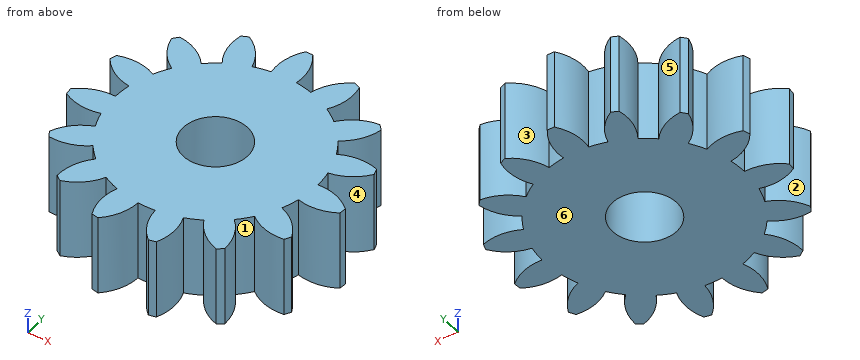
from build123d import *

# Parameters (mm, degrees)
MODEL_R             = 2
BOSS_EXTRUDE1_DEPTH = 5


with BuildPart() as part:
    # Model → Boss-Extrude1 (new body)
    with BuildSketch(Plane.XY):
        with BuildLine():
            ThreePointArc((455.213810884, 475.737053866), (455.579522306, 476.123501007), (455.911034715, 476.539656939))
            ThreePointArc((455.911034715, 476.539656939), (456.985627664, 475.992517671), (458.188848778, 475.912703304))
            ThreePointArc((458.188848778, 475.912703304), (458.297616539, 476.103235845), (458.401430664, 476.296512079))
            ThreePointArc((458.401430664, 476.296512079), (457.695483937, 477.274137059), (456.66162305, 477.894816565))
            ThreePointArc((456.66162305, 477.894816565), (456.838534846, 478.396601831), (456.972120634, 478.911617437))
            ThreePointArc((456.972120634, 478.911617437), (458.176351731, 478.848857172), (459.308012342, 479.265337237))
            ThreePointArc((459.308012342, 479.265337237), (459.329880069, 479.483637208), (459.346106466, 479.702428842))
            ThreePointArc((459.346106466, 479.702428842), (458.303556137, 480.3083993), (457.106624121, 480.454909137))
            ThreePointArc((457.106624121, 480.454909137), (457.064146634, 480.985269298), (456.976707605, 481.5100937))
            ThreePointArc((456.976707605, 481.5100937), (458.102354353, 481.942564259), (458.96678006, 482.783325568))
            ThreePointArc((458.96678006, 482.783325568), (458.897966625, 482.991646922), (458.823799602, 483.198122895))
            ThreePointArc((458.823799602, 483.198122895), (457.624912095, 483.327661034), (456.471869369, 482.974668319))
            ThreePointArc((456.471869369, 482.974668319), (456.217347342, 483.441899284), (455.9240025, 483.885785577))
            ThreePointArc((455.9240025, 483.885785577), (456.776430349, 484.73870887), (457.224154095, 485.858376156))
            ThreePointArc((457.224154095, 485.858376156), (457.076557966, 486.020698236), (456.924821674, 486.179156978))
            ThreePointArc((456.924821674, 486.179156978), (455.776895531, 485.809864476), (454.867113658, 485.018404858))
            ThreePointArc((454.867113658, 485.018404858), (454.444556262, 485.341718149), (453.996027593, 485.627914358))
            ThreePointArc((453.996027593, 485.627914358), (454.427844026, 486.753812201), (454.381450307, 487.958784817))
            ThreePointArc((454.381450307, 487.958784817), (454.180592196, 488.047040662), (453.977523219, 488.130083216))
            ThreePointArc((453.977523219, 488.130083216), (453.079045297, 487.325814102), (452.569833828, 486.232738138))
            ThreePointArc((452.569833828, 486.232738138), (452.052305076, 486.35622995), (451.526147262, 486.435250151))
            ThreePointArc((451.526147262, 486.435250151), (451.462687294, 487.639444578), (450.930198006, 488.721371813))
            ThreePointArc((450.930198006, 488.721371813), (450.710808105, 488.720301185), (450.491518914, 488.713568739))
            ThreePointArc((450.491518914, 488.713568739), (449.997844209, 487.613388449), (449.977250433, 486.407698904))
            ThreePointArc((449.977250433, 486.407698904), (449.454235747, 486.31001638), (448.941426255, 486.168197264))
            ThreePointArc((448.941426255, 486.168197264), (448.393662691, 487.242472118), (447.467150069, 488.014278923))
            ThreePointArc((447.467150069, 488.014278923), (447.267162884, 487.924066944), (447.069570573, 487.828723599))
            ThreePointArc((447.069570573, 487.828723599), (447.066059926, 486.622863301), (447.537644694, 485.51303485))
            ThreePointArc((447.537644694, 485.51303485), (447.099578065, 485.211068187), (446.688786314, 484.872931566))
            ThreePointArc((446.688786314, 484.872931566), (445.751432451, 485.631534965), (444.591098944, 485.959768933))
            ThreePointArc((444.591098944, 485.959768933), (444.445094078, 485.796014074), (444.303364151, 485.62854556))
            ThreePointArc((444.303364151, 485.62854556), (444.790624586, 484.525509454), (445.672846607, 483.703441519))
            ThreePointArc((445.672846607, 483.703441519), (445.395473735, 483.249403495), (445.157729351, 482.773416263))
            ThreePointArc((445.157729351, 482.773416263), (443.992862186, 483.085178789), (442.79934, 482.913085284))
            ThreePointArc((442.79934, 482.913085284), (442.732563019, 482.704102247), (442.67120187, 482.493465393))
            ThreePointArc((442.67120187, 482.493465393), (443.56498163, 481.683978441), (444.705296702, 481.291814037))
            ThreePointArc((444.705296702, 481.291814037), (444.636577876, 480.764211952), (444.612989023, 480.232676626))
            ThreePointArc((444.612989023, 480.232676626), (443.422024673, 480.043691705), (442.401684635, 479.401027258))
            ThreePointArc((442.401684635, 479.401027258), (442.425681887, 479.182951108), (442.455299415, 478.965566939))
            ThreePointArc((442.455299415, 478.965566939), (443.60105586, 478.589596791), (444.802293147, 478.695144705))
            ThreePointArc((444.802293147, 478.695144705), (444.954110477, 478.185205752), (445.148755882, 477.690029618))
            ThreePointArc((445.148755882, 477.690029618), (444.137622902, 477.03297446), (443.466891075, 476.030861592))
            ThreePointArc((443.466891075, 476.030861592), (443.577513216, 475.841399678), (443.692988281, 475.654855892))
            ThreePointArc((443.692988281, 475.654855892), (444.892609713, 475.777411201), (445.947064377, 476.36242124))
            ThreePointArc((445.947064377, 476.36242124), (446.293167267, 475.958318498), (446.67239097, 475.585122008))
            ThreePointArc((446.67239097, 475.585122008), (446.015923439, 474.573607419), (445.810775449, 473.385320549))
            ThreePointArc((445.810775449, 473.385320549), (445.988894907, 473.257232556), (446.170260821, 473.133784268))
            ThreePointArc((446.170260821, 473.133784268), (447.216321796, 473.733674108), (447.941669045, 474.696992722))
            ThreePointArc((447.941669045, 474.696992722), (448.422213161, 474.468599225), (448.92044394, 474.281911443))
            ThreePointArc((448.92044394, 474.281911443), (448.732151056, 473.090837485), (449.028058855, 471.921842207))
            ThreePointArc((449.028058855, 471.921842207), (449.242877156, 471.877275714), (449.458774107, 471.838268254))
            ThreePointArc((449.458774107, 471.838268254), (450.170401179, 472.811766221), (450.441221884, 473.986826871))
            ThreePointArc((450.441221884, 473.986826871), (450.973116782, 473.973633929), (451.504206009, 474.005734869))
            ThreePointArc((451.504206009, 474.005734869), (451.816645324, 472.84104905), (452.562443764, 471.893475269))
            ThreePointArc((452.562443764, 471.893475269), (452.776816874, 471.940136226), (452.989914315, 471.992314338))
            ThreePointArc((452.989914315, 471.992314338), (453.244060699, 473.171093791), (453.0135275, 474.354717814))
            ThreePointArc((453.0135275, 474.354717814), (453.504803721, 474.559006608), (453.976921244, 474.804345725))
            ThreePointArc((453.976921244, 474.804345725), (454.736069161, 473.867432804), (455.802802917, 473.305124634))
            ThreePointArc((455.802802917, 473.305124634), (455.979663777, 473.434944938), (456.153115226, 473.569286554))
            ThreePointArc((456.153115226, 473.569286554), (455.905836703, 474.749525816), (455.213810884, 475.737053866))
        make_face()
        with Locations((450.861979287, 480.22164557)):
            Circle(MODEL_R, mode=Mode.SUBTRACT)
    extrude(amount=BOSS_EXTRUDE1_DEPTH)


solid = part.part
Work out the finished part from the listing and answer in its coordinate system (mm). Face numbers are marked on the shaded views. A direction names the side the tool comes from. Give positions to 0.01 mm unless a question says otherwise; leave off trailing zeros. Order: outer loops, then holes, each group sorted by start corner. A loop starts at its lowest first (then second) coordinate and runs counter-clockwise, first axis right, second up. Notation, with made-up numbers: (17.5, -39) -> (22.5, -39) arc R24 cw to (22.5, -6) -> close; hole circle Ø6 at (-10, -1). An arc over 180 degrees is marked (long way). Answer as a JSON object with one key per item and string values. Group by question number.
1. Section A-A on y = 487.5 is taken. Determine the outline of the cut face in (x, z).
2. Section D-D on x = 453.5 is taken. Determine the outline of the cut face in (y, z).
3. Section C-C on y = 480 is taken. Determine the outline of the cut face in (x, z).
4. Flat-ended cylindrical pins translate along their axes: pin 1 Ø2 at (x, z) = (451.5, 2) entering from -Y; pin 2 Ø3 at (x, z) = (446.5, 3) entering from -Y; pin 3 Ø8 at (x, y) = (447, 477.5) entering from -Z. Find the tip coordinate at first contact, or state that the pin passes through.
5. Consider line 1 along Y through (x, z) = (450.75, 3.55); line 2 along X through (y, z) = (473.25, 3.1); line 3 along Y through (x, z) = (444, 0.3). Determine where each line is inside the solid, lowest interval first. Write a range as [from, to].
6. A tool of negligible diameter and unlimited length cuts with its end or side. For the marked faces 1, 2 and 3, from which of +Z, -Z, +X, -X, +Y, -Y can it reach the whole face along a straight path? Write none if from no direction.
7. The mould has two halves that part along X. Classify the marked faces 4, 5 and 6: released by +X, released by -X, zero draft, split by the parting line, or undercut.
8. Section B-B on x = 444 is taken. Determine the outline of the cut face in (y, z), plus the area to 3 significant figures.
Result sheet:
{
 "1": {"outline": "(447.02, 0) -> (448.16, 0) -> (448.16, 5) -> (447.02, 5) -> close; (449.97, 0) -> (451.5, 0) -> (451.5, 5) -> (449.97, 5) -> close; (453.22, 0) -> (454.46, 0) -> (454.46, 5) -> (453.22, 5) -> close"},
 "2": {"outline": "(474.56, 0) -> (487.78, 0) -> (487.78, 5) -> (474.56, 5) -> close"},
 "3": {"outline": "(443.31, 0) -> (448.87, 0) -> (448.87, 5) -> (443.31, 5) -> close; (452.85, 0) -> (458.95, 0) -> (458.95, 5) -> (452.85, 5) -> close"},
 "4": {"pin 1": "stops at y = 471.95", "pin 2": "stops at y = 473.13", "pin 3": "stops at z = 0"},
 "5": {"line 1": "y = [473.97, 478.22], [482.22, 488.72]", "line 2": "x = [446, 446.47], [448.73, 450.33], [451.65, 453.24]", "line 3": "y = [475.64, 476.89], [478.57, 480.2], [481.47, 483.08]"},
 "6": {"face 1": "+Z, -Z", "face 2": "+Z, -Z, -X", "face 3": "+Z, -Z, +Y"},
 "7": {"face 4": "released by +X", "face 5": "undercut", "face 6": "zero draft"},
 "8": {"outline": "(475.64, 0) -> (476.89, 0) -> (476.89, 5) -> (475.64, 5) -> close; (478.57, 0) -> (480.2, 0) -> (480.2, 5) -> (478.57, 5) -> close; (481.47, 0) -> (483.08, 0) -> (483.08, 5) -> (481.47, 5) -> close", "area": "22.4 mm^2"}
}
